Source: CAD feature listing. Evaluate the final solid. Frame: model axes, mm. Face numbers are marked on the shaded views. A direction names the side the tool comes from. Give positions to 0.01 mm unless a question says otherwise; leave off trailing zeros. Loops run counter-clockwise (first coordinate to the right, second up) from the corner with the lowest first, then second, coordinate; pieces in that order, holes last. Notation, with made-up numbers: M 19.5,12.5 L 68.5,12.5 A25 cw 68.5,29.5 Z; hole C -27,-9 d1. An arc over 180 degrees is marked long. Answer in a Markdown table with one row per item.
Autodesk Inventor part; units mm, degrees
ref_plane "YZ Plane" through (0, 0, 0) normal (1, 0, 0) x (0, 1, 0)
ref_plane "XZ Plane" through (0, 0, 0) normal (0, 1, 0) x (-1, 0, 0)
ref_plane "XY Plane" through (0, 0, 0) normal (0, 0, 1) x (1, 0, 0)
sketch "Sketch1" plane through (0, 0, 0) normal (0, 0, 1) x (1, 0, 0)
  circle A0 centre (0, 0) radius 10
  circle A1 centre (7, 0) radius 1.5
  circle A2 centre (0, 7) radius 1.5
  circle A3 centre (-7, 0) radius 1.5
  circle A4 centre (0, -7) radius 1.5
  circle A5 centre (0, 0) radius 1.5
  dimension "d0" = 20
  dimension "d1" = 3
  dimension "d2" = 7
  dimension "d5" = 360
  dimension "d7" = 3
extrude "Extrusion1" add sketch "Sketch1" along normal blind 2
sketch "Sketch2" plane through (0, 0, 2) normal (0, 0, 1) x (1, 0, 0)
  circle A0 centre (0, 0) radius 4.5
  circle A1 centre (0, 0) radius 1.5
  dimension "d10" = 9
extrude "Extrusion2" add sketch "Sketch2" along normal blind 3
sketch "Sketch3" plane through (0, 0, 5) normal (0, 0, 1) x (1, 0, 0)
  circle A0 centre (0, 0) radius 3
  dimension "d13" = 6
extrude "Extrusion3" cut sketch "Sketch3" against normal blind 3
properties part number "Servo Mounting Hub" material "Aluminum 6061"
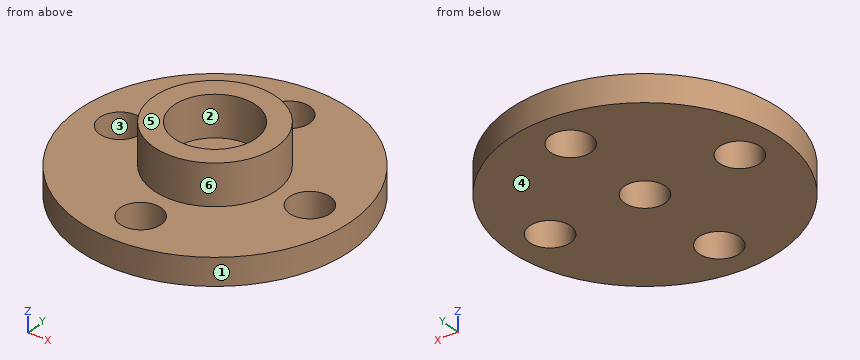
1) Section D-D, the plane y = 8. Return loops of the section in (x, z).
Reply:
| item | result |
|---|---|
| outline | M -6,0 L -1.12,0 L -1.12,2 L -6,2 Z; M 1.12,0 L 6,0 L 6,2 L 1.12,2 Z |
2) Section A-A, the plane x = 0. Return loops of the section in (y, z), then the cut area to 3 significant figures.
Reply:
| item | result |
|---|---|
| outline | M -10,0 L -8.5,0 L -8.5,2 L -10,2 Z; M -5.5,0 L -1.5,0 L -1.5,2 L -3,2 L -3,5 L -4.5,5 L -4.5,2 L -5.5,2 Z; M 1.5,0 L 5.5,0 L 5.5,2 L 4.5,2 L 4.5,5 L 3,5 L 3,2 L 1.5,2 Z; M 8.5,0 L 10,0 L 10,2 L 8.5,2 Z |
| area | 31.0 mm² |
3) Section B-B, the plane z = 1. Return loops of the section in (x, y), then the cut area to 3 significant figures.
Reply:
| item | result |
|---|---|
| outline | C 0,0 d20; hole C -7,0 d3; hole C 0,-7 d3; hole C 0,0 d3; hole C 0,7 d3; hole C 7,0 d3 |
| area | 279 mm² |
4) Set-up query: the marked faces 5 and 6. Return all of +Z, -Z, +X, -X, +Y, -Y with unobstructed straight access to the full face (end or side cutting, diameter ignored); none if empty.
Reply:
| item | result |
|---|---|
| face 5 | +Z, +X, -X, +Y, -Y |
| face 6 | +Z |
5) Pin query (flat end, axial travel): pin 1 Ø3 at (x, z) = (5, 4.5) entering from -Y; pin 2 Ø1 at (y, z) = (6, 1.5) entering from +X; pin 3 Ø1.5 at (x, z) = (-6.5, 2.5) entering from -Y; pin 4 Ø2.5 at (x, y) = (7, 0) entering from -Z. Return the tip coordinate at first contact, or that it passes through.
Reply:
| item | result |
|---|---|
| pin 1 | stops at y = -2.83 |
| pin 2 | stops at x = 8.35 |
| pin 3 | stops at y = -8.04 |
| pin 4 | passes through |
6) Pull-direction query (X, two-part tool) for the marked faces 1, 2, 3 and 4; classes: released by +X, released by -X, zero draft, split by the parting line, or undercut.
Reply:
| item | result |
|---|---|
| face 1 | split by the parting line |
| face 2 | undercut |
| face 3 | undercut |
| face 4 | zero draft |
7) Material intervals for L1, parallel to Y at x = 0, z = 1.45; L2, parallel to X at y = -0.25, z = 3.15; L3, parallel to Y at x = -1, z = 4, sorted ascending.
Reply:
| item | result |
|---|---|
| L1 | y = -10 to -8.5, -5.5 to -1.5, 1.5 to 5.5, 8.5 to 10 |
| L2 | x = -4.49 to -2.99, 2.99 to 4.49 |
| L3 | y = -4.39 to -2.83, 2.83 to 4.39 |
